Part model, mm, in its own coordinate system. A direction names the side the tool comes from. Round coordinates to 2 decimals unless told otherwise and drop trailing zeros. Write each loop counter-clockwise with the first axis right and the second up, starting at its lowest first coordinate (ties: lowest second). Pieces come first, ordered by that corner, then holes.
Autodesk Inventor part; units mm, degrees
ref_plane "YZ Plane" through (0, 0, 0) normal (1, 0, 0) x (0, 1, 0)
ref_plane "XZ Plane" through (0, 0, 0) normal (0, 1, 0) x (-1, 0, 0)
ref_plane "XY Plane" through (0, 0, 0) normal (0, 0, 1) x (1, 0, 0)
sketch "Sketch1" plane through (0, 0, 0) normal (0, 1, 0) x (-1, 0, 0)
  line L0 (-7.5, 30) -> (7.5, 30)
  line L1 (7.5, 30) -> (7.5, -21.5)
  line L2 (7.5, -21.5) -> (-7.5, -21.5)
  line L3 (-7.5, -21.5) -> (-7.5, 30)
  line L4 (7.5, -21.5) -> (47.5, -21.5)
  line L5 (47.5, -6.5) -> (7.5, -6.5)
  line L6 (47.5, -6.5) -> (47.5, -21.5)
  point P0 (0, 0)
  point P1 (0, -21.5)
  dimension "d30" = 15
  dimension "d31" = 21.5
  dimension "d32" = 30
  dimension "d61" = 15
  dimension "d91" = 40
extrude "Extrusion1" add sketch "Sketch1" along normal mid plane 3
sketch "Sketch4" plane through (0, 1.5, 0) normal (0, 1, 0) x (1, 0, 0)
  line L0 (7.5, 4.5) -> (-7.5, 4.5)
  line L1 (7.5, 4.5) -> (7.5, 14.5)
  line L2 (-7.5, 6.5) -> (-7.5, 4.5)
  line L3 (7.5, -30) -> (7.5, 21.5)
  line L4 (-7.5, 6.5) -> (-7.5, -30)
  line L5 (-7.5, -30) -> (7.5, -30)
  line L6 (7.5, 21.5) -> (-47.5, 21.5)
  line L7 (7.5, 21.5) -> (-7.5, 21.5)
  line L8 (-7.5, -30) -> (7.5, -30)
  line L9 (7.5, -30) -> (7.5, 21.5)
  line L10 (7.5, 21.5) -> (-47.5, 21.5)
  line L11 (-47.5, 6.5) -> (-7.5, 6.5)
  line L12 (-7.5, 6.5) -> (-7.5, -30)
  line L13 (-47.5, 21.5) -> (-47.5, 6.5)
  point P0 (0, 0)
  dimension "d89" = 2
extrude "Extrusion3" add sketch "Sketch4" along normal blind 3 contours L0 L2 L11 L13 L6 L3 L1
sketch "Sketch5" plane through (0, 1.5, 0) normal (0, 1, 0) x (1, 0, 0)
  line L0 (-2.5, -12) -> (-4.5, -12)
  line L1 (-4.5, -12) -> (-4.5, -2)
  line L2 (-4.5, -2) -> (-2.5, -2)
  line L3 (-2.5, -2) -> (-2.5, -12)
  line L4 (-2.5, -12) -> (-4.5, -2) construction
  line L5 (-4.5, -12) -> (-2.5, -2) construction
  line L6 (4.5, -12) -> (2.5, -12)
  line L7 (2.5, -12) -> (2.5, -2)
  line L8 (2.5, -2) -> (4.5, -2)
  line L9 (4.5, -2) -> (4.5, -12)
  line L10 (4.5, -12) -> (2.5, -2) construction
  line L11 (2.5, -12) -> (4.5, -2) construction
  line L12 (-3.5, -7) -> (3.5, -7) construction
  line L13 (-7.5, 4.5) -> (7.5, 4.5)
  point P0 (0, 0)
  point P1 (0, -7)
  dimension "d24" = 2
  dimension "d25" = 10
  dimension "d26" = 7
  dimension "d90" = 6.5
extrude "Extrusion4" cut sketch "Sketch5" against normal blind 2
sketch "Sketch6" plane through (0, 1.5, 0) normal (0, 1, 0) x (1, 0, 0)
  circle A0 centre (0, -18) radius 1.8986
  circle A1 centre (0, -26) radius 1.8986
  line L0 (1.8986, -26) -> (1.8986, -18)
  line L1 (-1.8986, -26) -> (-1.8986, -18)
  line L2 (-7.5, -30) -> (7.5, -30)
  point P0 (0, 0)
  dimension "d33" = 3.7973
  dimension "d36" = 3.7973
  dimension "d37" = 8
  dimension "d68" = 4
extrude "Extrusion5" cut sketch "Sketch6" against normal through all
fillet "Fillet2" radius 2 3 edges at (7.5, 1.5, -21.5) (7.5, 0, 30) (-7.5, 0, 30)
sketch "Sketch8" plane through (0, 1.5, 0) normal (0, 1, 0) x (1, 0, 0)
  line L0 (-7.5, 4.5) -> (7.5, 4.5)
  line L1 (-7.5, 4.5) -> (-7, 4.5)
  line L2 (-7, 4.5) -> (-7, 2.5)
  line L3 (-7, 2.5) -> (-7.5, 2.5)
  line L4 (-7.5, 2.5) -> (-7.5, 4.5)
  point P0 (0, 0)
  dimension "d74" = 0.5
  dimension "d75" = 2
extrude "Extrusion6" add sketch "Sketch8" along normal blind 1
sketch "Sketch10" plane through (0, 4.5, 0) normal (0, 1, 0) x (1, 0, 0)
  point P0 (0, 0)
sketch "Sketch11" plane through (0, 4.5, 0) normal (0, 1, 0) x (1, 0, 0)
  circle A0 centre (-27, 14) radius 1.8986
  circle A1 centre (-12, 14) radius 1.8987
  line L0 (-27, 12.1014) -> (-12, 12.1014)
  line L1 (-27, 15.8986) -> (-12, 15.8986)
  line L2 (-19.5, 6.5) -> (-19.5, 21.5) construction
  line L3 (5.5, 21.5) -> (-47.5, 21.5) construction
  line L4 (-47.5, 6.5) -> (-7.5, 6.5)
  line L5 (-7.5, 6.5) -> (-7.5, 4.5)
  point P0 (0, 0)
  point P1 (-19.5, 14)
  point P2 (-42.5, 21.5)
  point P3 (-19.5, 15.8986)
  dimension "d85" = 3.7973
  dimension "d86" = 15
  dimension "d92" = 12
extrude "Extrusion7" cut sketch "Sketch11" against normal blind 10
sketch "Sketch12" plane through (0, -1.5, 0) normal (0, 1, 0) x (1, 0, 0)
  circle A0 centre (-39.5, 14) radius 6.477
  line L0 (-47.5, 6.5) -> (-7.5, 6.5) construction
  line L1 (-39.5, 6.5) -> (-39.5, 21.5) construction
  line L2 (5.5, 21.5) -> (-47.5, 21.5) construction
  line L3 (-47.5, 6.5) -> (-47.5, 21.5) construction
  point P0 (0, 0)
  point P1 (-42.5, 21.5)
  point P2 (-47.5, 16.5)
  dimension "d93" = 12.954
  dimension "d96" = 8
extrude "Extrusion8" cut sketch "Sketch12" along normal blind 4.7625
fillet "Fillet3" radius 2 1 edges at (-47.5, 1.5, -6.5)
equation "\"d36\" = d33"
properties part number "FiberMount"
Q1. Cut at D-D on z = 9. Write the cut outline in (x, y).
Values follow:
outline: (-7.5, -1.5) - (7.5, -1.5) - (7.5, 1.5) - (4.5, 1.5) - (4.5, -0.5) - (2.5, -0.5) - (2.5, 1.5) - (-2.5, 1.5) - (-2.5, -0.5) - (-4.5, -0.5) - (-4.5, 1.5) - (-7.5, 1.5) - close
Q2. Cut at A-A on x = -21. Write the cut outline in (y, z), plus the area to 3 significant figures.
Values follow:
outline: (-1.5, -21.5) - (4.5, -21.5) - (4.5, -15.9) - (-1.5, -15.9) - close; (-1.5, -12.1) - (4.5, -12.1) - (4.5, -6.5) - (-1.5, -6.5) - close
area: 67.2 mm2
Q3. Which spindle directions (+Z, -Z, +X, -X, +Y, -Y) get a long thin tool onto all of the face, cutting with end or side? Do faces 5 (the flat face through (-27, 1, -6.5)), 6 (the cylindrical face through (0, 0, 16.1)), 7 (the flat face through (3, -0.5, 7)), 8 (the cylindrical face through (-33.322, 0.848, -12.054)). Say none if no direction does.
Values follow:
face 5: +Z, -X, +Y, -Y
face 6: +Y, -Y
face 7: +Y
face 8: -Y
Q4. Cut at B-B on z = -14. Write the cut outline in (x, y).
Values follow:
outline: (-47.5, -1.5) - (-45.98, -1.5) - (-45.98, 3.26) - (-33.02, 3.26) - (-33.02, -1.5) - (-28.9, -1.5) - (-28.9, 4.5) - (-47.5, 4.5) - close; (-10.1, -1.5) - (7.5, -1.5) - (7.5, 4.5) - (-10.1, 4.5) - close
Q5. Cut at C-C on x = 0. Write the cut outline in (y, z), plus the area to 3 significant figures.
Values follow:
outline: (-1.5, -21.5) - (4.5, -21.5) - (4.5, -4.5) - (1.5, -4.5) - (1.5, 16.1) - (-1.5, 16.1) - close; (-1.5, 27.9) - (1.5, 27.9) - (1.5, 30) - (-1.5, 30) - close
area: 170 mm2
Q6. Wall check: L1, parallel to X at y = 0.45, z = -14; L2, parallel to X at y = -0.35, z = 10; L3, parallel to Z at x = -39.5, y = -0.5. Give the ranges that are in metal, low to high.
Values follow:
L1: x = -47.5 to -45.98, -33.02 to -28.9, -10.1 to 7.5
L2: x = -7.5 to -4.5, -2.5 to 2.5, 4.5 to 7.5
L3: z = -21.5 to -20.48, -7.52 to -6.5
Q7. Drop flat-ended pins along their axis: pin 1 (0.6 mm diameter, centred on x = -3, z = 5.5, fed in from +Y); pin 2 (3.5 mm diameter, centred on y = 0.5, z = 21.5, fed in from -X); pin 3 (0.5 mm diameter, centred on y = 2, z = -3.5, fed in from +X). Give the stop position or say it passes through.
Values follow:
pin 1: stops at y = -0.5
pin 2: stops at x = -7.5
pin 3: stops at x = -7
Q8. Mould opens along Z. For faces 1 (the flat face through (-4, 1, 2)), 2 (the flat face through (2.5, 1, 7)), 3 (the flat face through (-47.5, 1, -15)), 4 (the cylindrical face through (-6.9, -0.02, 29.43)) say: +Z half, -Z half, draft (parallel to the pull), parting line (faces both ways), or undercut.
Values follow:
face 1: undercut
face 2: undercut
face 3: draft
face 4: +Z half
